The model under review builds one solid part; all positions refer to its coordinate system, in mm. A direction names the side the tool comes from. Round coordinates to 2 decimals unless told otherwise and drop trailing zeros. Order: outer loops, then holes, each group sorted by start corner. A loop starts at its lowest first (then second) coordinate and runs counter-clockwise, first axis right, second up. Notation, with made-up numbers: M -31.75,7 L 21.25,7 A31 cw 21.25,34 Z; hole C 20.25,87.25 d11. An arc over 180 degrees is marked long. Answer as a JSON object with one key per item and string values. Group by question number.
1) Consider section B-B, the plane z = 0. Write out the cut boundary in (x, y), then the cut area to 3 significant figures.
2) To check wall thickness, follow line 1 (X direction, y = 2.5, z = 34); line 2 (X direction, y = 1.25, z = 23); line 3 (Z direction, x = -8.5, y = 8.5). State the ranges of each line that lie inside material, in increasing order.
3) Insertion check: pin 1 Ø4 at (x, y) = (-56, 7.5) entering from +Z; pin 2 Ø1 at (y, z) = (2.5, -24) entering from -X; pin 3 Ø4 at (x, y) = (40.5, 8.5) entering from -Z. Each pin has a flat end and moves straight along its axis. Give the tip position at first contact, or say it passes through.
4) Consider section C-C, the plane x = 0. Write out the cut boundary in (y, z).
5) Consider section D-D, the plane x = -46. Write out the cut boundary in (y, z).
6) The part is to be moulded in two halves that separate along X. For faces 1 (the flat face through (85, 5, 86.6)), 2 (the cylindrical face through (10.4, 4.93, 80.95)), 3 (the cylindrical face through (-25.252, 4.93, -43.155)), say which applies: +X half, -X half, draft (parallel to the pull), parting line (faces both ways), or undercut.
7) Consider section A-A, the plane y = 8. Write out the cut boundary in (x, z).
8) For faces 4 (the cylindrical face through (-84.429, 4.93, -36.845)), 5 (the cylindrical face through (-24.748, 4.93, 43.446)), 6 (the cylindrical face through (81.65, 4.93, -62.14)), list the 3-axis set-ups (+Z, -Z, +X, -X, +Y, -Y) from which the entire face can be reached by the end or side of a thin tool; tool diameter is ignored.
```python
from build123d import *

# Parameters (mm, degrees)
IZIM1_R                     = 40
Y_KSEKLIK_EKSTR_ZYON1_DEPTH = 10


with BuildPart() as part:
    # Çizim1 → Yükseklik-Ekstrüzyon1 (new body)
    with BuildSketch(Plane(origin=(0, 0, 0), x_dir=(1, 0, 0), z_dir=(0, 1, 0))):
        with BuildLine():
            Line((-100, -40), (-100, -30))
            ThreePointArc((-100, -30), (-70, 0), (-100, 30))
            Line((-100, 30), (-100, 40))
            ThreePointArc((-100, 40), (-84.220237409, 36.755939555), (-71, 27.549954628))
            ThreePointArc((-71, 27.549954628), (-55.218260111, 21.366045629), (-40.357142857, 29.51780853))
            ThreePointArc((-40.357142857, 29.51780853), (-25.000226369, 43.301139494), (-5.38512036, 49.709158902))
            ThreePointArc((-5.38512036, 49.709158902), (9.104684892, 58.503090991), (11.64055433, 75.261881641))
            ThreePointArc((11.64055433, 75.261881641), (10.412263093, 80.871903754), (10, 86.6))
            Line((10, 86.6), (20, 86.6))
            ThreePointArc((20, 86.6), (50, 56.6), (80, 86.6))
            Line((80, 86.6), (90, 86.6))
            ThreePointArc((90, 86.6), (81.419623277, 61.845055583), (59.359636345, 47.710448608))
            ThreePointArc((59.359636345, 47.710448608), (46.113763964, 37.135262428), (45.742467512, 20.189766365))
            ThreePointArc((45.742467512, 20.189766365), (50, 0), (45.742467512, -20.189766365))
            ThreePointArc((45.742467512, -20.189766365), (46.113763964, -37.135262428), (59.359636345, -47.710448608))
            ThreePointArc((59.359636345, -47.710448608), (81.419623277, -61.845055583), (90, -86.6))
            Line((90, -86.6), (80, -86.6))
            ThreePointArc((80, -86.6), (50, -56.6), (20, -86.6))
            Line((20, -86.6), (10, -86.6))
            ThreePointArc((10, -86.6), (10.412263093, -80.871903754), (11.64055433, -75.261881641))
            ThreePointArc((11.64055433, -75.261881641), (9.104684892, -58.503090991), (-5.38512036, -49.709158902))
            ThreePointArc((-5.38512036, -49.709158902), (-25.000226369, -43.301139494), (-40.357142857, -29.51780853))
            ThreePointArc((-40.357142857, -29.51780853), (-55.218260111, -21.366045629), (-71, -27.549954628))
            ThreePointArc((-71, -27.549954628), (-84.220237409, -36.755939555), (-100, -40))
        make_face()
        with Locations(Location((0, 0, 0), (0, 0, 270))):
            Circle(IZIM1_R, mode=Mode.SUBTRACT)
    extrude(amount=Y_KSEKLIK_EKSTR_ZYON1_DEPTH)


solid = part.part
```
Results list:
{
 "1": {"outline": "M -70,0 L -40,0 L -40,10 L -70,10 Z; M 40,0 L 50,0 L 50,10 L 40,10 Z", "area": "400 mm^2"},
 "2": {"line 1": "-100 to -78.93, -36.66 to -21.07, 21.07 to 44.88", "line 2": "-80.74 to -64.51, -48.49 to -32.73, 32.73 to 44.75", "line 3": "-49.27 to -39.09, 39.09 to 49.27"},
 "3": {"pin 1": "z = 21.48", "pin 2": "x = -82.69", "pin 3": "z = -58.89"},
 "4": {"outline": "M 0,-51.07 L 10,-51.07 L 10,-40 L 0,-40 Z; M 0,40 L 10,40 L 10,51.07 L 0,51.07 Z"},
 "5": {"outline": "M 0,-24.3 L 10,-24.3 L 10,24.3 L 0,24.3 Z"},
 "6": {"face 1": "draft", "face 2": "-X half", "face 3": "undercut"},
 "7": {"outline": "M -100,-40 A40 ccw -71,-27.55 A20 cw -40.36,-29.52 A50 ccw -5.39,-49.71 A20 cw 11.64,-75.26 A40 ccw 10,-86.6 L 20,-86.6 A30 cw 80,-86.6 L 90,-86.6 A40 ccw 59.36,-47.71 A20 cw 45.74,-20.19 A50 ccw 45.74,20.19 A20 cw 59.36,47.71 A40 ccw 90,86.6 L 80,86.6 A30 cw 20,86.6 L 10,86.6 A40 ccw 11.64,75.26 A20 cw -5.39,49.71 A50 ccw -40.36,29.52 A20 cw -71,27.55 A40 ccw -100,40 L -100,30 A30 cw -100,-30 Z; hole C 0,0 d80"},
 "8": {"face 4": "-Z, +Y, -Y", "face 5": "+Z, +Y, -Y", "face 6": "+X, +Y, -Y"}
}
